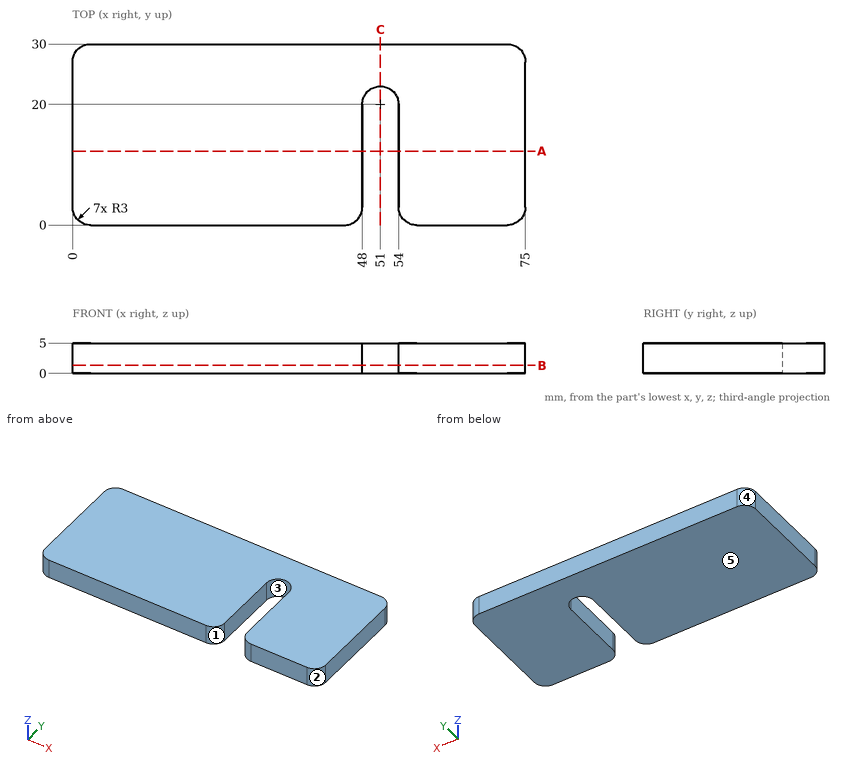
Check sheet for the drawn part. Datum: minimum x, y, z corner. Units: mm. A direction names the side the tool comes from. Round coordinates to 2 decimals unless told otherwise and drop trailing zeros. Order: outer loops, then holes, each group sorted by start corner. A loop starts at its lowest first (then second) coordinate and runs counter-clockwise, first axis right, second up. Notation, with made-up numbers: (67.5, 24.5) - (94.5, 24.5) arc R26 ccw to (94.5, 60.5) - close; hole circle Ø7 at (-19.75, 70.25). An arc over 180 degrees is marked (long way). Use a Markdown table: item, result. Add a question column.
(1) Material ranges on line 1 along X through (y, z) = (11.25, 0.7); line 2 along X through (y, z) = (1.75, 0.65); line 3 along Y through (x, z) = (50.5, 1.25), recorded low to high. Write a range as [from, to].
(2) Sectioned sample at B-B, the plane z = 1.3. Enter the section's corners in (x, y).
(3) Release check for a two-part mould opening along X. For the marked faces 3, 4 and 5 record: pulls with the +X half, pulls with the -X half, needs draft (parallel to the pull), parting line crosses it, or undercut.
(4) Sectioned sample at A-A, the plane y = 12.25. Enter the section's corners in (x, z), and give its area (3 significant figures).
(5) Sectioned sample at C-C, the plane x = 51. Enter the section's corners in (y, z), and give its area (3 significant figures).
(6) Tool access check on the marked faces 1 and 2. Record the directions out of +Z, -Z, +X, -X, +Y, -Y that give a thin tool (end or side, any length) a straight path to the whole face; none if there is none.
(7) Depth check by flat-ended pin: pin 1 (2 mm diameter, centred on x = 62, y = 3, fed in from -Z). Enter the tip coordinate at first touch or a pass-through.
Answers below:
| question | item | result |
|---|---|---|
| 1 | line 1 | [0, 48], [54, 75] |
| 1 | line 2 | [0.27, 47.73], [54.27, 74.73] |
| 1 | line 3 | [22.96, 30] |
| 2 | outline | (0, 3) arc R3 ccw to (3, 0) - (45, 0) arc R3 ccw to (48, 3) - (48, 20) arc R3 cw to (54, 20) - (54, 3) arc R3 ccw to (57, 0) - (72, 0) arc R3 ccw to (75, 3) - (75, 27) arc R3 ccw to (72, 30) - (3, 30) arc R3 ccw to (0, 27) - close |
| 3 | face 3 | undercut |
| 3 | face 4 | pulls with the -X half |
| 3 | face 5 | needs draft |
| 4 | outline | (0, 0) - (48, 0) - (48, 5) - (0, 5) - close; (54, 0) - (75, 0) - (75, 5) - (54, 5) - close |
| 4 | area | 345 mm² |
| 5 | outline | (23, 0) - (30, 0) - (30, 5) - (23, 5) - close |
| 5 | area | 35.0 mm² |
| 6 | face 1 | +Z, -Z, -Y |
| 6 | face 2 | +Z, -Z, +X, -Y |
| 7 | pin 1 | z = 0 |
